```python
from build123d import *

# Parameters (mm, degrees)
SKETCH_W        = 50
SKETCH_H        = 40
PAD_DEPTH       = 5.5
SKETCH004_W     = 3.5
SKETCH004_H     = 4.5
POCKET_DEPTH    = 5.501
SKETCH005_W     = 11
SKETCH005_H     = 14
POCKET001_DEPTH = 5.25
POCKET002_DEPTH = 4.5
SKETCH008_R     = 5
PAD001_DEPTH    = 20
SKETCH009_R     = 5
HOLE_DEPTH      = 20
FILLET_R        = 0.45
SKETCH010_W     = 37
SKETCH010_H     = 33.369954
POCKET003_DEPTH = 1.5
SKETCH012_R     = 2.95
PAD002_DEPTH    = 16


with BuildPart() as part:
    # Sketch → Pad (new body)
    with BuildSketch(Plane.XY):
        Rectangle(SKETCH_W, SKETCH_H)
    extrude(amount=PAD_DEPTH)

    # Sketch004 (on Face6 of Pad) → Pocket (cut, through all)
    with BuildSketch(Plane.XY.offset(5.5)):
        with Locations((-0.25, 0.25)):
            Rectangle(SKETCH004_W, SKETCH004_H)
    extrude(amount=-POCKET_DEPTH, mode=Mode.SUBTRACT)

    # Sketch005 (on Face5 of Pocket) → Pocket001 (cut)
    with BuildSketch(Plane.XY.offset(5.5)):
        with Locations((1.5, 0.3)):
            Rectangle(SKETCH005_W, SKETCH005_H)
    extrude(amount=-POCKET001_DEPTH, mode=Mode.SUBTRACT)

    # Sketch007 (on Face5 of Pocket001) → Pocket002 (cut)
    with BuildSketch(Plane.XY.offset(5.5)):
        with BuildLine():
            Line((-4, 8.05), (-2, 8.05))
            ThreePointArc((-2, 8.05), (-1.5, 7.550047), (-1, 8.05))
            Line((-1, 8.05), (4, 8.05))
            ThreePointArc((4, 8.05), (4.5, 7.54996), (5, 8.05))
            Line((5, 8.05), (7, 8.05))
            Line((7, 8.05), (7, -7.95))
            Line((7, -7.95), (4.999901, -7.95))
            ThreePointArc((4.999901, -7.95), (4.5, -7.459951), (4.000099, -7.95))
            Line((4.000099, -7.95), (-1, -7.95))
            ThreePointArc((-1, -7.95), (-1.5, -7.45043), (-2, -7.95))
            Line((-2, -7.95), (-4, -7.95))
            Line((-4, -7.95), (-4, 8.05))
        make_face()
    extrude(amount=-POCKET002_DEPTH, mode=Mode.SUBTRACT)

    # Sketch008 (on Face6 of Pocket002) → Pad001 (join)
    with BuildSketch(Plane.XZ.offset(20)):
        with Locations((25, 5.5)):
            Circle(SKETCH008_R)
    extrude(amount=-PAD001_DEPTH)

    # Sketch009 (on Face1 of Pad001) → Hole (cut)
    with BuildSketch(Plane(origin=(0, 20, 0), x_dir=(-1, 0, 0), z_dir=(0, 1, 0))):
        with Locations((-25, 5.5)):
            Circle(SKETCH009_R)
    extrude(amount=-HOLE_DEPTH, mode=Mode.SUBTRACT)

    # Fillet
    fillet_edges = [part.edges().sort_by_distance(p)[0] for p in [
        (25, 0, 0),
    ]]
    fillet(fillet_edges, radius=FILLET_R)

    # Sketch010 (on Face6 of Fillet) → Pocket003 (cut)
    with BuildSketch(Plane.XY.offset(5.5)):
        with Locations((-2.5, 0.684977)):
            Rectangle(SKETCH010_W, SKETCH010_H)
    extrude(amount=-POCKET003_DEPTH, mode=Mode.SUBTRACT)

    # Sketch012 (on Face22 of Pocket003) → Pad002 (join)
    with BuildSketch(Plane(origin=(0, 0, 0), x_dir=(-1, 0, 0), z_dir=(0, 1, 0))):
        with Locations((-25.000006, 5.5)):
            Circle(SKETCH012_R)
    extrude(amount=PAD002_DEPTH)


solid = part.part
```
Model file for the job. Use its own axes, mm. A direction names the side the tool comes from. Give positions to 0.01 mm unless a question says otherwise; leave off trailing zeros. Loops run counter-clockwise (first coordinate to the right, second up) from the corner with the lowest first, then second, coordinate; pieces in that order, holes last. Notation, with made-up numbers: (56, 83) -> (107, 83) arc R19 cw to (107, 98) -> close; hole circle Ø6 at (-6.75, -2). An arc over 180 degrees is marked (long way). Use CSV: the item, a comma, the result in double quotes. Start each with the question number.
1) Flat gauge pins, fed straight in: pin 1 Ø16.5 at (x, y) = (6, -5) entering from +Z; pin 2 Ø12 at (x, y) = (11.5, -1.5) entering from +Z. Where does each tip first touch, or does it go through?
2) Tool access for faces 1 (the flat face through (27, 0, 3)), 2 (the flat face through (2, -7, 1)), 3 (the flat face through (-25, 0, 3)): list every direction of +Z, -Z, +X, -X, +Y, -Y with a clear straight run to the whole face (end or side of a thin tool).
3) Slice it at A-A on y = 5. Give the cut face in (x, z), plus the area to 3 significant figures.
4) Slice it at B-B on x = 11.5. Give the cut face in (y, z), plus the area to 3 significant figures.
5) Slice it at C-C on y = -17. Give the cut face in (x, z).
6) Wall check: line 1 (Z direction, x = 2, y = -2.5); line 2 (Z direction, x = -16, y = -10.5); line 3 (Y direction, x = 1, z = 0.75). Give the ranges that are in metal, low to high.
7) Mould opens along Y. For faces 4 (the cylindrical face through (22.186, 7.888, 6.386)), 5 (the flat face through (-4, 0, 2)), 6 (the flat face through (25, 16, 6)) say: released by +Y, released by -Y, zero draft, split by the parting line, or undercut.
Computed values:
1,pin 1,"stops at z = 4"
1,pin 2,"stops at z = 5.5"
2,face 1,"+Y"
2,face 2,"+Z"
2,face 3,"+Z, -Z, -X, +Y, -Y"
3,outline,"(-25, 0) -> (24.55, 0) arc R0.45 ccw to (25, 0.45) -> (25, 0.5) arc R5 cw to (20, 5.5) -> (16, 5.5) -> (16, 4) -> (7, 4) -> (7, 0.25) -> (-4, 0.25) -> (-4, 4) -> (-21, 4) -> (-21, 5.5) -> (-25, 5.5) -> close; circle Ø5.9 at (25, 5.5)"
3,area,"186 mm^2"
4,outline,"(-20, 0) -> (20, 0) -> (20, 5.5) -> (17.37, 5.5) -> (17.37, 4) -> (-16, 4) -> (-16, 5.5) -> (-20, 5.5) -> close"
4,area,"170 mm^2"
5,outline,"(-25, 0) -> (24.55, 0) arc R0.45 ccw to (25, 0.45) -> (25, 0.5) arc R5 ccw (long way) to (20, 5.5) -> (-25, 5.5) -> close"
6,line 1,"z = 0 to 0.25"
6,line 2,"z = 0 to 4"
6,line 3,"y = -20 to -6.7, 7.3 to 20"
7,face 4,"zero draft"
7,face 5,"undercut"
7,face 6,"released by +Y"
